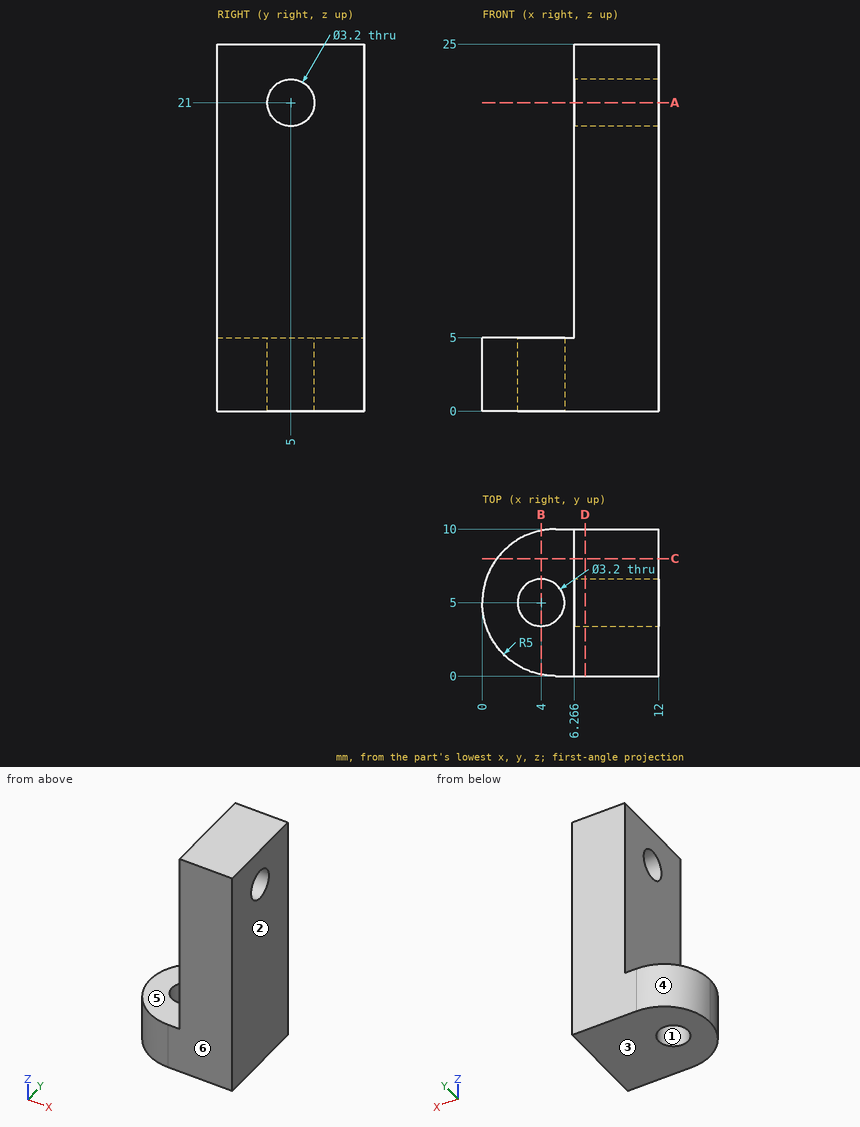
Could you check a few things on this drawing? It's one solid part, dimensions in mm from its lowest x, y, z. A direction names the side the tool comes from. Round coordinates to 2 decimals unless told otherwise and drop trailing zeros. Loops run counter-clockwise (first coordinate to the right, second up) from the corner with the lowest first, then second, coordinate; pieces in that order, holes last. Notation, with made-up numbers: M -37.5,2.25 L 6.5,2.25 A29 ccw 6.5,35.25 Z; hole C -28,80.5 d4. An arc over 180 degrees is marked long. Write each question's results on one line, items separated by ' | '. Start each with the question number.
(1) I want a section at B-B (x = 4). Please give me the cut outline in (y, z).
(2) I want a section at D-D (x = 7). Please give me the cut outline in (y, z).
(3) Thinking about a two-plate mould opening in X: for the marked faces 1, 2, 3 and 4, which applies, pulls with the +X half, pulls with the -X half, needs draft (parallel to the pull), parting line crosses it, or undercut?
(4) On a 3-axis mill with a long thin cutter (end or side, diameter ignored), from which of +Z, -Z, +X, -X, +Y, -Y can I reach the whole of each face in a straight line? I mean the marked faces 5 and 6. Say none if no direction works.
(5) I want a section at C-C (y = 8). Please give me the cut outline in (x, z), then the cut area to 3 significant figures.
(6) If I drill on probe 1 along Z at (x, y) = (7.5, 5); probe 2 along X at (y, z) = (6.75, 5.5); probe 3 along Z at (x, y) = (6, 5.25), over which ranges is the centre line in solid material (lowest first)? Write a range as from..to.
(7) Will these pins go through, and if not, where does the flat tip stop? P1, Ø5, axis at y = 5, z = 21, coming from the +X side; P2, Ø4, axis at x = 4, z = 10.5, coming from the +Y side; P3, Ø5, axis at y = 4.5, z = 11.5, coming from the -X side.
(8) I want a section at A-A (z = 21). Please give me the cut outline in (x, y), then the cut area to 3 significant figures.
Solved:
1) outline: M 0.1,0 L 3.4,0 L 3.4,5 L 0.1,5 Z; M 6.6,0 L 9.9,0 L 9.9,5 L 6.6,5 Z
2) outline: M 0,0 L 10,0 L 10,25 L 0,25 Z; hole C 5,21 d3.2
3) face 1: undercut | face 2: pulls with the +X half | face 3: needs draft | face 4: pulls with the -X half
4) face 5: +Z, -X, +Y, -Y | face 6: +Z, -Z, +X, -X, -Y
5) outline: M 1,0 L 12,0 L 12,25 L 6.27,25 L 6.27,5 L 1,5 Z | area: 170 mm²
6) probe 1: z = 0..19.4, 22.6..25 | probe 2: x = 6.27..12 | probe 3: z = 0..5
7) P1: stops at x = 12 | P2: passes through | P3: stops at x = 6.27
8) outline: M 6.27,0 L 12,0 L 12,3.4 L 6.27,3.4 Z; M 6.27,6.6 L 12,6.6 L 12,10 L 6.27,10 Z | area: 39.0 mm²
